Autodesk Inventor part; units mm, degrees
ref_plane "YZ Plane" through (0, 0, 0) normal (1, 0, 0) x (0, 1, 0)
ref_plane "XZ Plane" through (0, 0, 0) normal (0, 1, 0) x (-1, 0, 0)
ref_plane "XY Plane" through (0, 0, 0) normal (0, 0, 1) x (1, 0, 0)
sketch "Sketch1" plane through (0, 0, 0) normal (0, 1, 0) x (-1, 0, 0)
  line L0 (-17.5, -17.5) -> (17.5, 17.5) construction
  line L1 (17.5, -17.5) -> (-17.5, 17.5) construction
  circle A0 centre (15, -15) radius 2.05
  circle A1 centre (-15, -15) radius 2.05
  circle A2 centre (-15, 15) radius 2.05
  circle A3 centre (15, 15) radius 2.05
  line L2 (20, 20) -> (-20, 20)
  line L3 (-20, 20) -> (-20, -20)
  line L4 (-20, -20) -> (20, -20)
  line L5 (20, -20) -> (20, 20)
  line L6 (20, 20) -> (-20, -20) construction
  line L7 (-20, 20) -> (20, -20) construction
  circle A4 centre (12, 0) radius 3.05
  circle A5 centre (-12, 0) radius 3.05
  point P0 (0, 0)
  dimension "d0" = 35
  dimension "d1" = 35
  dimension "d2" = 4.1
  dimension "d3" = 4.1
  dimension "d4" = 4.1
  dimension "d5" = 4.1
  dimension "d6" = 30
  dimension "d7" = 30
  dimension "d8" = 30
  dimension "d9" = 30
  dimension "d10" = 40
  dimension "d11" = 40
  dimension "d14" = 6.1
  dimension "d15" = 8
  dimension "d16" = 6.1
  dimension "d17" = 8
extrude "Extrusion2" add sketch "Sketch1" along normal blind 5
sketch "Sketch2" plane through (20, 0, 20) normal (1, 0, 0) x (0, 0, -1)
  circle A0 centre (20, 2.5) radius 1
  line L0 (0, 5) -> (40, 5)
  point P0 (20, 0)
  dimension "d20" = 2
  dimension "d21" = 2.5
hole "Hole1" at (20, 2.5, 0) direction (-1, 0, 0) diameter 2 depth 8 tip angle 118
thread "Thread1"
sketch "Sketch3" plane through (-20, 0, -20) normal (-1, 0, 0) x (0, 0, 1)
  circle A0 centre (20, 2.5) radius 1
  circle A1 centre (20, 2.5) radius 1
  point P0 (20, 0)
  dimension "d31" = 2
hole "Hole2" at (-20, 2.5, 0) direction (1, 0, 0) diameter 2 depth 8 tip angle 118
thread "Thread2"
sketch "Sketch4" plane through (0, 5, 0) normal (0, 1, 0) x (1, 0, 0)
  line L0 (7, -9) -> (-7, -9)
  line L1 (-7, -9) -> (-7, 9)
  line L2 (-7, 9) -> (7, 9)
  line L3 (7, 9) -> (7, -9)
  line L4 (7, -9) -> (-7, 9) construction
  line L5 (-7, -9) -> (7, 9) construction
  point P0 (0, 0)
  dimension "d41" = 14
  dimension "d42" = 18
extrude "Extrusion3" cut sketch "Sketch4" against normal blind 10
fillet "Fillet1" radius 2 1 edges at (20, 2.5, 20)
fillet "Fillet2" radius 2 1 edges at (20, 2.5, -20)
fillet "Fillet3" radius 2 1 edges at (-20, 2.5, -20)
fillet "Fillet4" radius 2 1 edges at (-20, 2.5, 20)
fillet "Fillet5" radius 2 1 edges at (-7, 2.5, -9)
fillet "Fillet6" radius 2 1 edges at (-7, 2.5, 9)
fillet "Fillet7" radius 2 1 edges at (7, 2.5, -9)
fillet "Fillet8" radius 2 1 edges at (7, 2.5, 9)
properties part number "AdapterPlate"
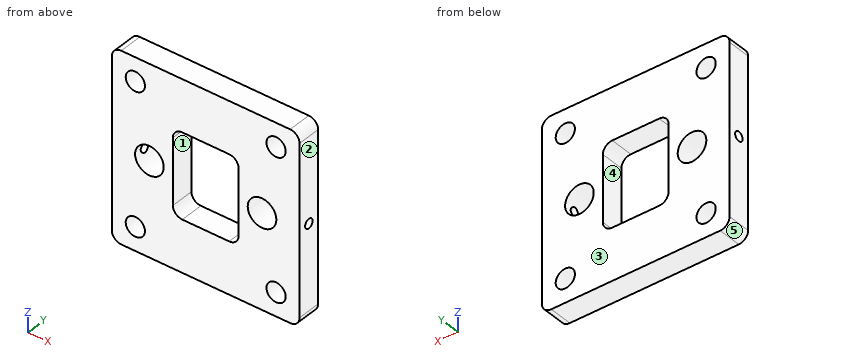
Build history of the part. All positions in model axes, mm. Face numbers are marked on the shaded views. A direction names the side the tool comes from. Round coordinates to 2 decimals unless told otherwise and drop trailing zeros. Write each loop counter-clockwise with the first axis right and the second up, starting at its lowest first coordinate (ties: lowest second). Pieces come first, ordered by that corner, then holes. Notation, with made-up numbers: (-21.5, -3.5) - (-14.5, -3.5) arc R22 cw to (-14.5, 3.5) - close; hole circle Ø1 at (-32, 1.5). An arc over 180 degrees is marked (long way). One line per question, with ' | ' between items.
1. Tool access for the marked faces 1 and 2: list every direction of +Z, -Z, +X, -X, +Y, -Y with a clear straight run to the whole face (end or side of a thin tool).
Results are:
face 1: +Y, -Y | face 2: +Z, -Z, +X, +Y, -Y
2. Mould opens along X. For the marked faces 3, 4 and 5 say: released by +X, released by -X, zero draft, split by the parting line, or undercut.
Results are:
face 3: zero draft | face 4: undercut | face 5: released by -X
3. Band-saw the part on B-B, the plane z = 0. Write the cut outline in (x, y), and give its area (3 significant figures).
Results are:
outline: (-20, 0) - (-15.05, 0) - (-15.05, 1.5) - (-20, 1.5) - close; (-20, 3.5) - (-15.05, 3.5) - (-15.05, 5) - (-20, 5) - close; (-8.95, 0) - (-7, 0) - (-7, 5) - (-8.95, 5) - close; (7, 0) - (8.95, 0) - (8.95, 5) - (7, 5) - close; (15.05, 0) - (20, 0) - (20, 1.5) - (15.05, 1.5) - close; (15.05, 3.5) - (20, 3.5) - (20, 5) - (15.05, 5) - close | area: 49.2 mm^2
4. Drop flat-ended pins along their axis: pin 1 Ø1.6 at (y, z) = (2.5, 0) entering from -X; pin 2 Ø1.2 at (y, z) = (2.5, 0) entering from -X. Give the stop position or say it passes through.
Results are:
pin 1: x = -9.06 | pin 2: x = -9.01
5. Band-saw the part on D-D, the plane z = -15. Write the cut outline in (x, y), and give its area (3 significant figures).
Results are:
outline: (-20, 0) - (-17.05, 0) - (-17.05, 5) - (-20, 5) - close; (-12.95, 0) - (12.95, 0) - (12.95, 5) - (-12.95, 5) - close; (17.05, 0) - (20, 0) - (20, 5) - (17.05, 5) - close | area: 159 mm^2
6. Band-saw the part on A-A, the plane x = 3. Write the cut outline in (y, z), and give its area (3 significant figures).
Results are:
outline: (0, -20) - (5, -20) - (5, -9) - (0, -9) - close; (0, 9) - (5, 9) - (5, 20) - (0, 20) - close | area: 110 mm^2
7. Drill centre lines: line 1 along Z through (x, y) = (16.85, 2.5); line 2 along Z through (x, y) = (-15, 3.1); line 3 along X through (y, z) = (2.55, -5). Where is each one in solid material? Low to high. Write a range as from..to.
Results are:
line 1: -20..-15.88, -14.12..-1, 1..14.12, 15.88..20 | line 2: -20..-17.05, -12.95..-0.8, 0.8..12.95, 17.05..20 | line 3: -20..-7, 7..20
8. Band-saw the part on C-C, the plane y = 2.5. Write the cut outline in (x, z), and give its area (3 significant figures).
Results are:
outline: (-20, -18) arc R2 ccw to (-18, -20) - (18, -20) arc R2 ccw to (20, -18) - (20, -1) - (14.88, -1) arc R3.05 cw (long way) to (14.88, 1) - (20, 1) - (20, 18) arc R2 ccw to (18, 20) - (-18, 20) arc R2 ccw to (-20, 18) - (-20, 1) - (-14.88, 1) arc R3.05 cw (long way) to (-14.88, -1) - (-20, -1) - close; hole circle Ø4.1 at (-15, -15); hole circle Ø4.1 at (-15, 15); hole (-7, -7) arc R2 ccw to (-5, -9) - (5, -9) arc R2 ccw to (7, -7) - (7, 7) arc R2 ccw to (5, 9) - (-5, 9) arc R2 ccw to (-7, 7) - close; hole circle Ø4.1 at (15, -15); hole circle Ø4.1 at (15, 15) | area: 1,220 mm^2
